Can you work these out from the model? Positions are in its coordinate system, mm. Give positions to 0.01 mm unless a question says otherwise; leave off trailing zeros. Write each loop counter-clockwise with the first axis right and the second up, starting at its lowest first coordinate (ties: lowest second). Pieces come first, ordered by that corner, then holes. Notation, with made-up numbers: (-30.5, -28.5) -> (-22.5, -28.5) arc R16 ccw to (-22.5, -5.5) -> close; hole circle Ø9 at (22, 14). An arc over 180 degrees is marked (long way). One line per item, written item: value.
from build123d import *

# Parameters (mm, degrees)
DODANIE_WYCI_GNI_CIE1_DEPTH = 10
SZKIC2_R                    = 1.75
DODANIE_WYCI_GNI_CIE2_DEPTH = 12


with BuildPart() as part:
    # Szkic1 → Dodanie-wyciągnięcie1 (new body)
    with BuildSketch(Plane.XY):
        with BuildLine():
            Line((1.75, 0), (1.75, 19.5))
            Line((1.75, 19.5), (-1.75, 19.5))
            Line((-1.75, 19.5), (-1.75, 5.5))
            ThreePointArc((-1.75, 5.5), (0.277964608, 3.903301802), (-0.798314607, 1.557303371))
            ThreePointArc((-0.798314607, 1.557303371), (-0.912537517, -1.493243209), (1.75, 0))
        make_face()
    extrude(amount=DODANIE_WYCI_GNI_CIE1_DEPTH)

    # Szkic2 → Dodanie-wyciągnięcie2 (add)
    with BuildSketch(Plane(origin=(0, 0, 0), x_dir=(-1, 0, 0), z_dir=(0, 0, -1))):
        Circle(SZKIC2_R)
    extrude(amount=-DODANIE_WYCI_GNI_CIE2_DEPTH)


solid = part.part
1) If we section it at A-A (x = 0): Write out the boundary of the cut face in (y, z), and give its area (3 significant figures).
Answer list:
outline: (-1.75, 0) -> (2.28, 0) -> (2.28, 10) -> (1.75, 10) -> (1.75, 12) -> (-1.75, 12) -> close; (4.55, 0) -> (19.5, 0) -> (19.5, 10) -> (4.55, 10) -> close
area: 197 mm^2
2) If we section it at B-B (x = 1.3): Write out the boundary of the cut face in (y, z), and give its area (3 significant figures).
Answer list:
outline: (-1.17, 0) -> (19.5, 0) -> (19.5, 10) -> (1.17, 10) -> (1.17, 12) -> (-1.17, 12) -> close
area: 211 mm^2
3) If we section it at D-D (y = 16): Write out the boundary of the cut face in (x, z), and give its area (3 significant figures).
Answer list:
outline: (-1.75, 0) -> (1.75, 0) -> (1.75, 10) -> (-1.75, 10) -> close
area: 35.0 mm^2
4) I need wall thicknesses on L1, parallel to Z at x = -0.6, y = 11; L2, parallel to Y at x = -0.9, z = 3; L3, parallel to Y at x = -0.55, z = 4.25. Which ranges of each line are inside material? Lowest first, please.
Answer list:
L1: z = 0 to 10
L2: y = -1.5 to 1.5, 5.32 to 19.5
L3: y = -1.66 to 1.71, 5.12 to 19.5
5) If we section it at C-C (z = 5): Write out the boundary of the cut face in (x, y).
Answer list:
outline: (-1.75, 5.5) arc R2.09 cw to (-0.8, 1.56) arc R1.75 ccw (long way) to (1.75, 0) -> (1.75, 19.5) -> (-1.75, 19.5) -> close
